```python
from build123d import *

# Parameters (mm, degrees)
SKETCH4_RX          = 1.9685
SKETCH4_RY          = 1.54305
BOSS_EXTRUDE2_DEPTH = 5.08
BOSS_EXTRUDE3_DEPTH = 0.508
SKETCH6_R           = 0.635
CUT_EXTRUDE2_DEPTH  = 27.625210039


# Read off the part's stored shape, not the designer's step: Boss-Extrude3
with BuildPart() as part:
    # Sketch3 → Revolve1 (revolve)
    with BuildSketch(Plane(origin=(0, 0, 0), x_dir=(-1, 0, 0), z_dir=(0, 1, 0))):
        with BuildLine():
            Line((-25.908, 0), (25.908, 0))
            ThreePointArc((25.908, 0), (25.372399433, -1.217244883), (24.113105869, -1.644717447))
            Line((24.113105869, -1.644717447), (18.288, -1.135086719))
            Line((18.288, -1.135086719), (18.288, -0.6985))
            Line((18.288, -0.6985), (5.5245, -0.6985))
            Line((5.5245, -0.6985), (5.5245, -1.3335))
            ThreePointArc((5.5245, -1.3335), (0, -2.54), (-5.5245, -1.3335))
            Line((-5.5245, -1.3335), (-5.5245, -0.6985))
            Line((-5.5245, -0.6985), (-18.288, -0.6985))
            Line((-18.288, -0.6985), (-18.288, -1.135086719))
            Line((-18.288, -1.135086719), (-24.113105869, -1.644717447))
            ThreePointArc((-24.113105869, -1.644717447), (-25.372399433, -1.217244883), (-25.908, 0))
        make_face()
    revolve(axis=Axis((25.908, 0, 0), (-1, 0, 0)))

    # Sketch4 → Boss-Extrude2 (add)
    with BuildSketch(Plane(origin=(0, 0, 0), x_dir=(-1, 0, 0), z_dir=(0, 1, 0))):
        with Locations((0, 0)):
            Ellipse(SKETCH4_RX, SKETCH4_RY)
    extrude(amount=BOSS_EXTRUDE2_DEPTH)

    # Boss-Extrude3 outline → Boss-Extrude3 (add)
    with BuildSketch(Plane(origin=(0, 5.08, 0), x_dir=(-1, 0, 0), z_dir=(0, 1, 0))):
        with BuildLine():
            add(Edge.make_bspline(
                [(2.7305, 0), (2.7305, 0.328264155), (2.559294063, 0.984792465), (1.681563155, 1.991576732), (0, 2.514032178), (-1.681563155, 1.991576732), (-2.559294063, 0.984792465), (-2.816102969, 0), (-2.559294063, -0.984792465), (-1.681563155, -1.991576732), (0, -2.514032178), (1.681563155, -1.991576732), (2.559294063, -0.984792465), (2.7305, -0.328264155), (2.7305, 0)],
                knots=[0, 0, 0, 0, 0.392699082, 0.785398163, 1.570796327, 2.35619449, 2.748893572, 3.141592654, 3.534291735, 3.926990817, 4.71238898, 5.497787144, 5.890486225, 6.283185307, 6.283185307, 6.283185307, 6.283185307], degree=3))
        make_face()
    extrude(amount=BOSS_EXTRUDE3_DEPTH)

    # Sketch6 → Cut-Extrude2 (cut, through all)
    with BuildSketch(Plane(origin=(0, 0, 0), x_dir=(-1, 0, 0), z_dir=(0, 1, 0))):
        with Locations(Location((0, 0, 0), (0, 0, 90))):
            Circle(SKETCH6_R)
    extrude(amount=CUT_EXTRUDE2_DEPTH, mode=Mode.SUBTRACT)


solid = part.part
```
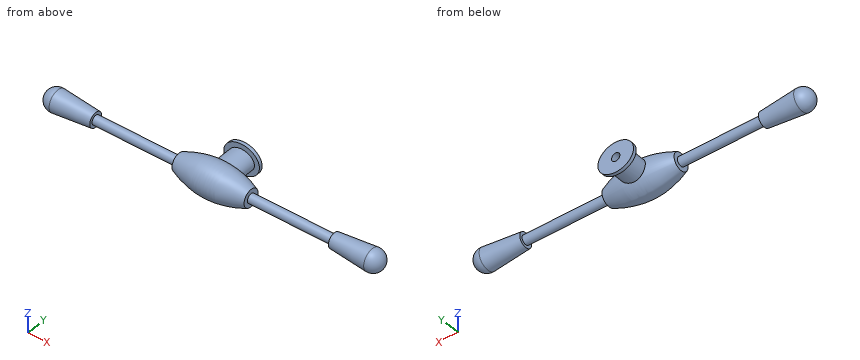
The listing builds one solid part. Answer for the finished solid, in the listing's coordinates (mm). Give positions to 0.01 mm unless a question says otherwise; leave off trailing zeros. Order: outer loops, then holes, each group sorted by start corner. A loop starts at its lowest first (then second) coordinate and runs counter-clockwise, first axis right, second up.
1) Find section B-B on x = 19. Write down the section's boundary in (y, z).
Reported:
outline: circle Ø2.39 at (0, 0)
2) Given P1, Ø1, axis at x = -16.5, z = -1, coming from the -Y side; P2, Ø1.4, axis at x = -1, z = 0.5, coming from the -Y side; P3, Ø1.5, axis at y = 3, z = 1.5, coming from the +X side, each flat-ended and moving along its own axis, determine where each tip first touches the part or whether it passes through.
Reported:
P1: stops at y = -0.49
P2: stops at y = -2.53
P3: stops at x = 1.72
3) Find section A-A on x = -17.5. Write down the section's boundary in (y, z).
Reported:
outline: circle Ø1.4 at (0, 0)
4) Consider line 1 along Z through (x, y) = (0, 3.7) (3 decimals); line 2 along X through (y, z) = (0, -1); line 3 along X through (y, z) = (5, 0.35). Determine where each line is inside the solid, lowest interval first.
Reported:
line 1: z = -1.543 to -0.635, 0.635 to 1.543
line 2: x = -25.57 to -18.29, -5.52 to 5.52, 18.29 to 25.57
line 3: x = -1.92 to -0.53, 0.53 to 1.92
